Verification items for the finished model (mm, model axes). A direction names the side the tool comes from. Round coordinates to 2 decimals unless told otherwise and drop trailing zeros. Order: outer loops, then holes, each group sorted by start corner. A loop starts at its lowest first (then second) coordinate and runs counter-clockwise, first axis right, second up. Notation, with made-up numbers: M 42.25,80 L 86.25,80 A23 ccw 86.25,92 Z; hole C -12,-14.5 d9. An arc over 180 degrees is marked long. One line per item, written item: value. Start each with the question number.
from build123d import *

# Parameters (mm, degrees)
SKETCH1_W           = 186
SKETCH1_H           = 95
BOSS_EXTRUDE1_DEPTH = 5
SKETCH2_W           = 150
SKETCH2_H           = 60
CUT_EXTRUDE1_DEPTH  = 1
SKETCH4_R           = 1.75
BOSS_EXTRUDE2_DEPTH = 186
SKETCH6_W           = 96.969797672
SKETCH6_H           = 5
BOSS_EXTRUDE3_DEPTH = 2
BOSS_EXTRUDE4_START = 5
SKETCH7_R           = 1.75
BOSS_EXTRUDE4_DEPTH = 5


with BuildPart() as part:
    # Sketch1 → Boss-Extrude1 (new body)
    with BuildSketch(Plane(origin=(0, 0, 0), x_dir=(1, 0, 0), z_dir=(0, 1, 0))):
        Rectangle(SKETCH1_W, SKETCH1_H)
    extrude(amount=BOSS_EXTRUDE1_DEPTH)

    # Sketch2 → Cut-Extrude1 (cut)
    with BuildSketch(Plane(origin=(0, 5, 0), x_dir=(1, 0, 0), z_dir=(0, 1, 0))):
        with Locations((0, -8.418340883)):
            Rectangle(SKETCH2_W, SKETCH2_H)
    extrude(amount=-CUT_EXTRUDE1_DEPTH, mode=Mode.SUBTRACT)

    # Sketch4 → Boss-Extrude2 (add, through all)
    with BuildSketch(Plane.ZY.offset(93)):
        with BuildLine():
            Line((-47.5, 0), (-47.5, 5))
            Line((-47.5, 5), (-54.5, 5))
            ThreePointArc((-54.5, 5), (-57, 2.5), (-54.5, 0))
            Line((-54.5, 0), (-47.5, 0))
        make_face()
        with Locations((-54.5, 2.5)):
            Circle(SKETCH4_R, mode=Mode.SUBTRACT)
    extrude(amount=-BOSS_EXTRUDE2_DEPTH)

    # Sketch6 → Boss-Extrude3 (add)
    with BuildSketch(Plane.ZY.offset(93)):
        with Locations((-0.984898836, 2.5)):
            Rectangle(SKETCH6_W, SKETCH6_H)
    boss_extrude3 = extrude(amount=BOSS_EXTRUDE3_DEPTH)

    # Mirror2: Boss-Extrude3 across plane
    add(boss_extrude3.mirror(Plane.ZY))

    # Sketch7 → Boss-Extrude4 (add)
    with BuildSketch(Plane.ZY.offset(95).offset(BOSS_EXTRUDE4_START)):
        with BuildLine():
            Line((-54.5, 5), (47.5, 5))
            Line((47.5, 5), (47.5, 0))
            Line((47.5, 0), (-54.5, 0))
            ThreePointArc((-54.5, 0), (-57, 2.5), (-54.5, 5))
        make_face()
        with Locations((-54.5, 2.5)):
            Circle(SKETCH7_R, mode=Mode.SUBTRACT)
    boss_extrude4 = extrude(amount=-BOSS_EXTRUDE4_DEPTH)

    # Mirror3: Boss-Extrude4 across plane
    add(boss_extrude4.mirror(Plane.ZY))


solid = part.part
1. Section check B-B (x = 53). Record the cut outline in (y, z), and give its area (3 significant figures).
2. Scan lines: line 1 along X through (y, z) = (4.3, -7.5); line 2 along Y through (x, z) = (-98.7, -54.5); line 3 along Y through (x, z) = (-42, -20). Record each from-to range of solid material in increasing order.
3. Tool access check on faces 4 (the face through (95, 3, -52)), 5 (the face through (100, 3, -4)), 6 (the face through (-1, 4, 8)). Record the directions out of +Z, -Z, +X, -X, +Y, -Y that give a thin tool (end or side, any length) a straight path to the whole face; none if there is none.
4. Draft check along Z on faces 1 (the face through (97.5, 2.4, -57)), 2 (the face through (-100, 3, -4)), 3 (the face through (-1.302, 1.83, -52.883)). Enter one of: released by +Z, released by -Z, zero draft, split by the parting line, or undercut.
5. Depth check by flat-ended pin: pin 1 (3 mm diameter, centred on y = 2.5, z = -54.5, fed in from -X); pin 2 (0.6 mm diameter, centred on x = 93.5, y = 2, fed in from -Z); pin 3 (18 mm diameter, centred on x = 9, z = -4.5, fed in from +Y); pin 4 (2 mm diameter, centred on x = -94.5, y = 1.5, fed in from -Z). Enter the tip coordinate at first touch or a pass-through.
6. Section check C-C (z = -1). Record the cut outline in (x, y), and give its area (3 significant figures).
7. Section check D-D (x = -79). Record the cut outline in (y, z).
8. Section check A-A (y = 2.5). Record the cut outline in (x, z).
Geometry check:
1. outline: M 0,-54.5 A2.5 ccw 5,-54.5 L 5,-21.58 L 4,-21.58 L 4,38.42 L 5,38.42 L 5,47.5 L 0,47.5 Z; hole C 2.5,-54.5 d3.5
1. area: 450 mm²
2. line 1: x = -100 to -75, 75 to 100
2. line 2: y = 0 to 0.75, 4.25 to 5
2. line 3: y = 0 to 4
3. face 4: -Z, +Y, -Y
3. face 5: +Z, -Z, +X, +Y, -Y
3. face 6: +Y
4. face 1: released by -Z
4. face 2: zero draft
4. face 3: undercut
5. pin 1: passes through
5. pin 2: stops at z = -49.47
5. pin 3: stops at y = 4
5. pin 4: stops at z = -57
6. outline: M -100,0 L 100,0 L 100,5 L 75,5 L 75,4 L -75,4 L -75,5 L -100,5 Z
6. area: 850 mm²
7. outline: M 0,-54.5 A2.5 ccw 5,-54.5 L 5,47.5 L 0,47.5 Z; hole C 2.5,-54.5 d3.5
8. outline: M -100,-57 L -95,-57 L -95,-56.25 L -100,-56.25 Z; M -100,-52.75 L -95,-52.75 L -95,-49.47 L -93,-49.47 L -93,-52.75 L 93,-52.75 L 93,-49.47 L 95,-49.47 L 95,-52.75 L 100,-52.75 L 100,47.5 L -100,47.5 Z; M -93,-57 L 93,-57 L 93,-56.25 L -93,-56.25 Z; M 95,-57 L 100,-57 L 100,-56.25 L 95,-56.25 Z
